Geometry: final body of the model. Coordinates: model frame, mm. Face numbers are marked on the shaded views. A direction names the side the tool comes from. Coordinates: 2 decimals unless noted, no trailing zeros. Loops run counter-clockwise (first coordinate to the right, second up) from the corner with the lowest first, then second, coordinate; pieces in that order, holes last. Notation, with made-up numbers: (2.5, 13) - (61.5, 13) arc R26 cw to (61.5, 40) - close; hole circle Ø8 at (85, 8.5). An arc over 180 degrees is marked (long way). Answer in a Markdown table with one row per item.
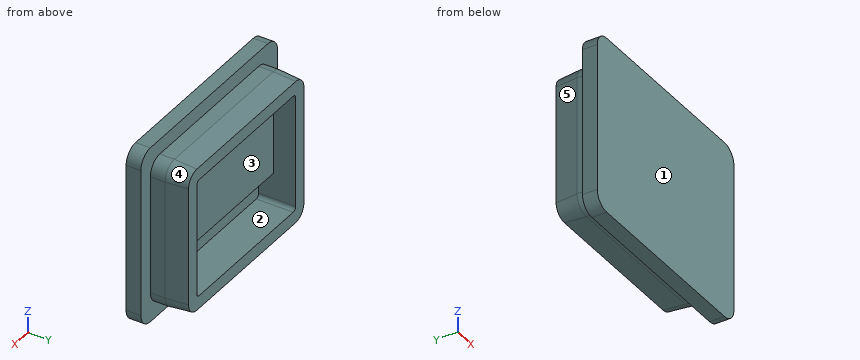
from build123d import *
from OCP.BRepFilletAPI import BRepFilletAPI_MakeChamfer

# Parameters (mm, degrees)
SKETCH1_W           = 29
SKETCH1_H           = 24
BOSS_EXTRUDE1_DEPTH = 2
SKETCH2_W           = 25
SKETCH2_H           = 20
SKETCH2_W_2         = 21
SKETCH2_H_2         = 16
BOSS_EXTRUDE2_DEPTH = 5
SKETCH3_W           = 21
SKETCH3_H           = 12
SKETCH3_R           = 0.975
BOSS_EXTRUDE3_DEPTH = 2
FILLET1_R           = 2
FILLET5_R           = 0.5
CHAMFER1_SIZE       = 3
CHAMFER1_SIZE2      = 0.262465991


with BuildPart() as part:
    # Sketch1 → Boss-Extrude1 (new body)
    with BuildSketch(Plane(origin=(0, 0, 0), x_dir=(1, 0, 0), z_dir=(0, 1, 0))):
        Rectangle(SKETCH1_W, SKETCH1_H)
    extrude(amount=BOSS_EXTRUDE1_DEPTH)

    # Sketch2 → Boss-Extrude2 (add)
    with BuildSketch(Plane(origin=(0, 2, 0), x_dir=(1, 0, 0), z_dir=(0, 1, 0))):
        Rectangle(SKETCH2_W, SKETCH2_H)
        Rectangle(SKETCH2_W_2, SKETCH2_H_2, mode=Mode.SUBTRACT)
    extrude(amount=BOSS_EXTRUDE2_DEPTH)

    # Sketch3 → Boss-Extrude3 (add)
    with BuildSketch(Plane(origin=(0, 2, 0), x_dir=(1, 0, 0), z_dir=(0, 1, 0))):
        with Locations((0, -2)):
            Rectangle(SKETCH3_W, SKETCH3_H)
        with Locations(Location((-7.5, -5.3, 0), (0, 0, 270))):
            Circle(SKETCH3_R, mode=Mode.SUBTRACT)
        with Locations(Location((7.5, -5.3, 0), (0, 0, 90))):
            Circle(SKETCH3_R, mode=Mode.SUBTRACT)
    extrude(amount=BOSS_EXTRUDE3_DEPTH)

    # Fillet1
    fillet1_edges = [part.edges().sort_by_distance(p)[0] for p in [
        (-12.5, 4.5, -10),
        (-12.5, 4.5, 10),
        (12.5, 4.5, 10),
        (12.5, 4.5, -10),
        (14.5, 1, 12),
        (-14.5, 1, 12),
        (-14.5, 1, -12),
        (14.5, 1, -12),
    ]]
    fillet(fillet1_edges, radius=FILLET1_R)

    # Fillet5
    fillet5_edges = [part.edges().sort_by_distance(p)[0] for p in [
        (10.5, 4.5, -8),
        (-10.5, 4.5, -8),
        (-10.5, 5.5, 8),
        (10.5, 5.5, 8),
    ]]
    fillet(fillet5_edges, radius=FILLET5_R)

    # Chamfer1: one chamfer whose edges measure the first distance from different faces: ONE call of the kernel's chamfer builder (chamfer() names one face for all edges)
    chamfer1_edges_1 = [part.edges().sort_by_distance(p)[0] for p in [
        (0, 7, -10),
    ]]
    chamfer1_side_1 = [part.faces().sort_by_distance(p)[0] for p in [
        (0, 4.5, -10),
    ]]
    chamfer1_edges_2 = [part.edges().sort_by_distance(p)[0] for p in [
        (12.5, 7, 0),
    ]]
    chamfer1_side_2 = [part.faces().sort_by_distance(p)[0] for p in [
        (12.5, 4.5, 0),
    ]]
    chamfer1_edges_3 = [part.edges().sort_by_distance(p)[0] for p in [
        (-12.5, 7, 0),
    ]]
    chamfer1_side_3 = [part.faces().sort_by_distance(p)[0] for p in [
        (-12.5, 4.5, 0),
    ]]
    chamfer1_edges_4 = [part.edges().sort_by_distance(p)[0] for p in [
        (0, 7, 10),
    ]]
    chamfer1_side_4 = [part.faces().sort_by_distance(p)[0] for p in [
        (0, 4.5, 10),
    ]]
    chamfer1_edges_5 = [part.edges().sort_by_distance(p)[0] for p in [
        (-11.914213562, 7, -9.414213562),
    ]]
    chamfer1_side_5 = [part.faces().sort_by_distance(p)[0] for p in [
        (-11.914213562, 4.5, -9.414213562),
    ]]
    chamfer1_edges_6 = [part.edges().sort_by_distance(p)[0] for p in [
        (-11.914213562, 7, 9.414213562),
    ]]
    chamfer1_side_6 = [part.faces().sort_by_distance(p)[0] for p in [
        (-11.914213562, 4.5, 9.414213562),
    ]]
    chamfer1_edges_7 = [part.edges().sort_by_distance(p)[0] for p in [
        (11.914213562, 7, 9.414213562),
    ]]
    chamfer1_side_7 = [part.faces().sort_by_distance(p)[0] for p in [
        (11.914213562, 4.5, 9.414213562),
    ]]
    chamfer1_edges_8 = [part.edges().sort_by_distance(p)[0] for p in [
        (11.914213562, 7, -9.414213562),
    ]]
    chamfer1_side_8 = [part.faces().sort_by_distance(p)[0] for p in [
        (11.914213562, 4.5, -9.414213562),
    ]]
    chamfer1 = BRepFilletAPI_MakeChamfer(part.part.solid().wrapped)
    for e in chamfer1_edges_1:
        chamfer1.Add(CHAMFER1_SIZE, CHAMFER1_SIZE2, e.wrapped, chamfer1_side_1[0].wrapped)  # the first distance lies on this face
    for e in chamfer1_edges_2:
        chamfer1.Add(CHAMFER1_SIZE, CHAMFER1_SIZE2, e.wrapped, chamfer1_side_2[0].wrapped)  # the first distance lies on this face
    for e in chamfer1_edges_3:
        chamfer1.Add(CHAMFER1_SIZE, CHAMFER1_SIZE2, e.wrapped, chamfer1_side_3[0].wrapped)  # the first distance lies on this face
    for e in chamfer1_edges_4:
        chamfer1.Add(CHAMFER1_SIZE, CHAMFER1_SIZE2, e.wrapped, chamfer1_side_4[0].wrapped)  # the first distance lies on this face
    for e in chamfer1_edges_5:
        chamfer1.Add(CHAMFER1_SIZE, CHAMFER1_SIZE2, e.wrapped, chamfer1_side_5[0].wrapped)  # the first distance lies on this face
    for e in chamfer1_edges_6:
        chamfer1.Add(CHAMFER1_SIZE, CHAMFER1_SIZE2, e.wrapped, chamfer1_side_6[0].wrapped)  # the first distance lies on this face
    for e in chamfer1_edges_7:
        chamfer1.Add(CHAMFER1_SIZE, CHAMFER1_SIZE2, e.wrapped, chamfer1_side_7[0].wrapped)  # the first distance lies on this face
    for e in chamfer1_edges_8:
        chamfer1.Add(CHAMFER1_SIZE, CHAMFER1_SIZE2, e.wrapped, chamfer1_side_8[0].wrapped)  # the first distance lies on this face
    add(Compound.cast(chamfer1.Shape()), mode=Mode.REPLACE)


solid = part.part
(1) Cut plane B-B on z = 1.75. Output: boundary loops of the cut face in (x, y).
Verdict:
| item | result |
|---|---|
| outline | (-14.5, 0) - (14.5, 0) - (14.5, 2) - (12.5, 2) - (12.5, 4) - (12.24, 7) - (10.5, 7) - (10.5, 4) - (-10.5, 4) - (-10.5, 7) - (-12.24, 7) - (-12.5, 4) - (-12.5, 2) - (-14.5, 2) - close |
(2) Cut plane A-A on x = -5.25. Output: boundary loops of the cut face in (y, z).
Verdict:
| item | result |
|---|---|
| outline | (0, -12) - (2, -12) - (2, -10) - (4, -10) - (7, -9.74) - (7, -8) - (2, -8) - (2, -4) - (4, -4) - (4, 8) - (7, 8) - (7, 9.74) - (4, 10) - (2, 10) - (2, 12) - (0, 12) - close |
(3) First-contact query: pin 1 Ø1.2 at (x, z) = (7.5, 5.3) entering from +Y; pin 2 Ø1.5 at (y, z) = (5, 0) entering from -X; pin 3 Ø6 at (x, z) = (0.5, -0.5) entering from +Y. Flat tips, straight axial feed; report the tip coordinate or a pass-through.
Verdict:
| item | result |
|---|---|
| pin 1 | stops at y = 2 |
| pin 2 | stops at x = -12.48 |
| pin 3 | stops at y = 4 |
(4) Pull-direction query (Z, two-part tool) for the marked faces 3, 4 and 5; classes: pulls with the +Z half, pulls with the -Z half, needs draft (parallel to the pull), parting line crosses it, or undercut.
Verdict:
| item | result |
|---|---|
| face 3 | undercut |
| face 4 | pulls with the +Z half |
| face 5 | needs draft |
(5) Cut plane C-C on z = 5.3. Output: boundary loops of the cut face in (x, y) (3 decimals), then the cut area to 3 significant figures.
Verdict:
| item | result |
|---|---|
| outline | (-14.5, 0) - (14.5, 0) - (14.5, 2) - (12.5, 2) - (12.5, 4) - (12.238, 7) - (10.5, 7) - (10.5, 4) - (8.475, 4) - (8.475, 2) - (6.525, 2) - (6.525, 4) - (-6.525, 4) - (-6.525, 2) - (-8.475, 2) - (-8.475, 4) - (-10.5, 4) - (-10.5, 7) - (-12.238, 7) - (-12.5, 4) - (-12.5, 2) - (-14.5, 2) - close |
| area | 111 mm² |
(6) Ray query, probe 1 along X at (y, z) = (2.6, 5.3) (3 decimals); probe 2 along Z at (x, y) = (7.5, 3.5) (3 decimals); probe 3 along X at (y, z) = (4, -5.25). Return the intervals inside material, ascending.
Verdict:
| item | result |
|---|---|
| probe 1 | x = -12.5 to -8.475, -6.525 to 6.525, 8.475 to 12.5 |
| probe 2 | z = -10 to -8, -4 to 4.325, 6.275 to 10 |
| probe 3 | x = -12.5 to -10.5, 10.5 to 12.5 |
(7) Access query for the marked faces 1 and 2. Directions: +Z, -Z, +X, -X, +Y, -Y. A direction counts if a zero-diameter tool reaches every point of the face in a straight line with its end or side. Return the directions, or none.
Verdict:
| item | result |
|---|---|
| face 1 | +Z, -Z, +X, -X, -Y |
| face 2 | +Y |
